Here's the drawing with two shaded views (mm, measured from the low corner). I have some questions. Coordinates: 2 decimals unless noted, no trailing zeros. Write each loop counter-clockwise with the first axis right and the second up, starting at its lowest first coordinate (ties: lowest second). Pieces come first, ordered by that corner, then holes.
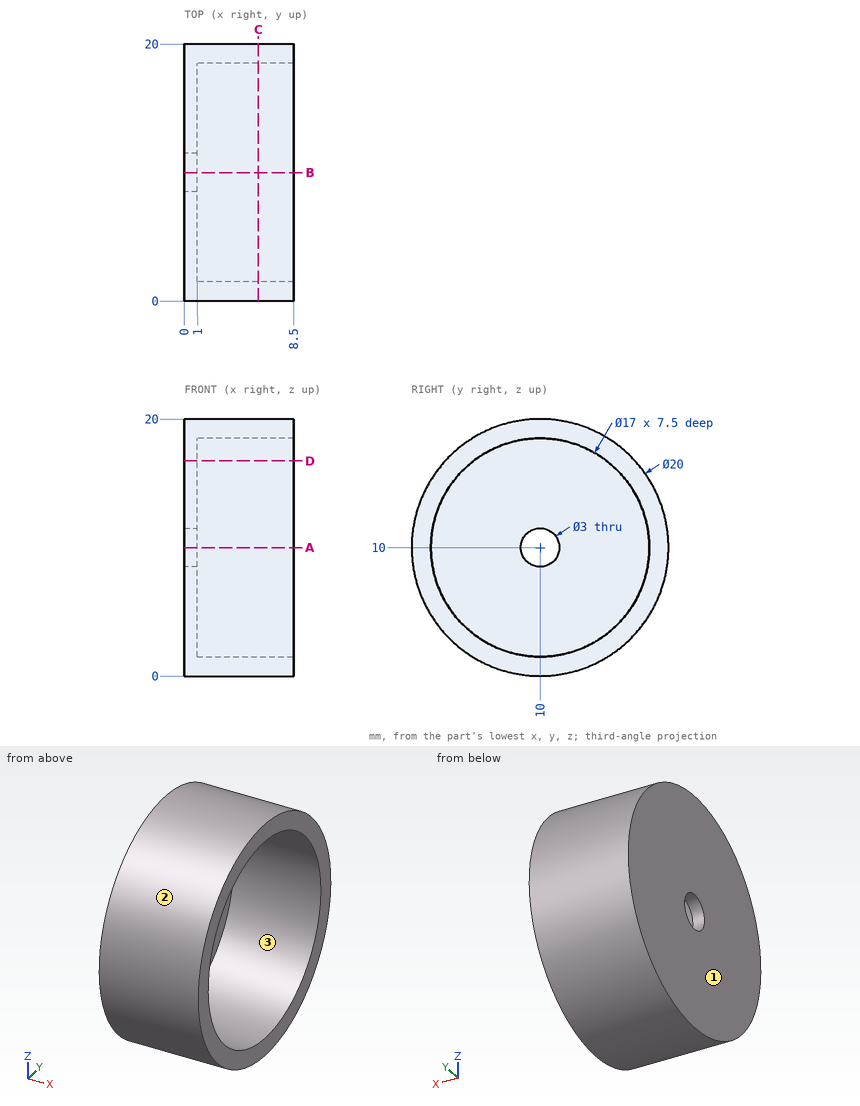
Item 1: If I drill on line 1 along Y through (x, z) = (2.5, 10); line 2 along Y through (x, z) = (0.65, 10); line 3 along X through (y, z) = (14, 13.25), over which ranges is the centre line in solid material (lowest first)?
Item 2: I want a section at C-C, the plane x = 5.75. List the corners of the cut face in (y, z) for me.
Item 3: I want a section at A-A, the plane z = 10. List the corners of the cut face in (x, y) for me.
Item 4: If we mould it in two halves opening along Z, with no side actions, what happens to the marked faces 1, 2 and 3? For each: released by +Z, released by -Z, zero draft, split by the parting line, or undercut.
Item 5: Will these pins go through, and if not, where does the flat tip stop? pin 1 Ø1 at (y, z) = (13.5, 9.5) entering from +X; pin 2 Ø3 at (x, y) = (3, 18) entering from -Z; pin 3 Ø1 at (x, z) = (1, 17) entering from +Y.
Item 6: I want a section at D-D, the plane z = 16.75. List the corners of the cut face in (x, y) for me.
Taken from the geometry:
1. line 1: y = 0 to 1.5, 18.5 to 20
1. line 2: y = 0 to 8.5, 11.5 to 20
1. line 3: x = 0 to 1
2. outline: circle Ø20 at (10, 10); hole circle Ø17 at (10, 10)
3. outline: (0, 0) - (8.5, 0) - (8.5, 1.5) - (1, 1.5) - (1, 8.5) - (0, 8.5) - close; (0, 11.5) - (1, 11.5) - (1, 18.5) - (8.5, 18.5) - (8.5, 20) - (0, 20) - close
4. face 1: zero draft
4. face 2: split by the parting line
4. face 3: undercut
5. pin 1: stops at x = 1
5. pin 2: stops at z = 2.4
5. pin 3: stops at y = 17.6
6. outline: (0, 2.62) - (8.5, 2.62) - (8.5, 4.83) - (1, 4.83) - (1, 15.17) - (8.5, 15.17) - (8.5, 17.38) - (0, 17.38) - close
